from build123d import *

# Parameters (mm, degrees)
SKETCH1_R             = 5.715
BOSS_EXTRUDE1_DEPTH   = 76.2
SKETCH4_R             = 5.715
SKETCH4_R_2           = 5.207
BOSS_EXTRUDE2_DEPTH   = 3.81
F_6_32_TAPPED_HOLE1_D = 2.7051


with BuildPart() as part:
    # Sketch1 → Boss-Extrude1 (new body)
    with BuildSketch(Plane(origin=(0, 0, 0), x_dir=(1, 0, 0), z_dir=(0, 1, 0))):
        with BuildLine():
            Line((0, 8.255), (-10.795, 8.255))
            Line((-10.795, 8.255), (-10.795, -8.255))
            Line((-10.795, -8.255), (0, -8.255))
            ThreePointArc((0, -8.255), (8.255, 0), (0, 8.255))
        make_face()
        with Locations(Location((0, 0, 0), (0, 0, 90))):
            Circle(SKETCH1_R, mode=Mode.SUBTRACT)
    extrude(amount=BOSS_EXTRUDE1_DEPTH)

    # Sketch4 → Boss-Extrude2 (add)
    with BuildSketch(Plane.XZ):
        with Locations(Location((0, 0, 0), (0, 0, 270))):
            Circle(SKETCH4_R)
        with Locations(Location((0, 0, 0), (0, 0, 270))):
            Circle(SKETCH4_R_2, mode=Mode.SUBTRACT)
    extrude(amount=-BOSS_EXTRUDE2_DEPTH)

    # #6-32 Tapped Hole1 (through all)
    with Locations(Plane.ZY.offset(10.795)):
        with Locations((0, 69.85)):
            Hole(F_6_32_TAPPED_HOLE1_D / 2)


solid = part.part
The model under review builds one solid part; all positions refer to its coordinate system, in mm. A direction names the side the tool comes from. Give positions to 0.01 mm unless a question says otherwise; leave off trailing zeros. Order: outer loops, then holes, each group sorted by start corner. A loop starts at its lowest first (then second) coordinate and runs counter-clockwise, first axis right, second up. Notation, with made-up numbers: M -25.5,72.25 L 21.5,72.25 A12 cw 21.5,78.25 Z; hole C 3.5,4.25 d3. An arc over 180 degrees is marked long. Answer in a Markdown table with one row per item. Add a question column.
1. Add section B-B on y = 12. State the section outline as (x, z) points (3 decimals), plus the area to 3 significant figures.
2. Add section C-C on x = -1.25. State the section outline as (y, z) points (3 decimals), plus the area to 3 significant figures.
3. To check wall thickness, follow line 1 along X through (y, z) = (58.5, 0) (3 decimals); line 2 along Y through (x, z) = (-7, 0); line 3 along X through (y, z) = (1.3, 0) (3 decimals). State the ranges of each line that lie inside material, in increasing order.
4. Mouldability with a two-part tool opening along Z and no side actions: class faces 1 (the cylindrical face through (-5.666, 39.498, 0.744)), 2 (the flat face through (-5, 38, -8.255)), 3 (the flat face through (-5.4, 0, 0.1)) as released by +Z, released by -Z, zero draft, split by the parting line, or undercut.
5. Machinability: for faces 4 (the flat face through (-6, 76.2, -2)), 5 (the flat face through (-5, 3.81, -2)), which of the approach directions +Z, -Z, +X, -X, +Y, -Y give a long, thin tool a straight path to every point of the face, cutting with its end or side? Answer none if there is none.
6. Add section A-A on z = 0. State the section outline as (x, y) points (3 decimals).
7. Add section D-D on y = 69.85. State the section outline as (x, z) points (3 decimals).
8. For pin 1 Ø4 at (y, z) = (56.5, -4) entering from +X; pin 2 Ø6 at (x, z) = (0, 0) entering from -Y, all flat-tipped, find the tip position at first contact; note any pin that passes through.
The answers:
| question | item | result |
|---|---|---|
| 1 | outline | M -10.795,-8.255 L 0,-8.255 A8.255 ccw 0,8.255 L -10.795,8.255 Z; hole C 0,0 d11.43 |
| 1 | area | 183 mm2 |
| 2 | outline | M 0,-8.255 L 76.2,-8.255 L 76.2,-5.577 L 3.81,-5.577 L 3.81,-5.055 L 0,-5.055 Z; M 0,5.055 L 3.81,5.055 L 3.81,5.577 L 76.2,5.577 L 76.2,8.255 L 0,8.255 Z |
| 2 | area | 412 mm2 |
| 3 | line 1 | -10.795 to -5.715, 5.715 to 8.255 |
| 3 | line 2 | 0 to 68.5, 71.2 to 76.2 |
| 3 | line 3 | -10.795 to -5.207, 5.207 to 8.255 |
| 4 | face 1 | undercut |
| 4 | face 2 | released by -Z |
| 4 | face 3 | zero draft |
| 5 | face 4 | +Z, -Z, +X, -X, +Y |
| 5 | face 5 | +Y |
| 6 | outline | M -10.795,0 L -5.207,0 L -5.207,3.81 L -5.715,3.81 L -5.715,68.497 L -10.795,68.497 Z; M -10.795,71.203 L -5.715,71.203 L -5.715,76.2 L -10.795,76.2 Z; M 5.207,0 L 8.255,0 L 8.255,68.497 L 5.715,68.497 L 5.715,3.81 L 5.207,3.81 Z; M 5.715,71.203 L 8.255,71.203 L 8.255,76.2 L 5.715,76.2 Z |
| 7 | outline | M -10.795,-8.255 L 0,-8.255 A8.255 ccw 8.143,-1.353 L 5.553,-1.353 A5.715 cw -5.553,-1.353 L -10.795,-1.353 Z; M -10.795,1.353 L -5.553,1.353 A5.715 cw 5.553,1.353 L 8.143,1.353 A8.255 ccw 0,8.255 L -10.795,8.255 Z |
| 8 | pin 1 | x = 8.01 |
| 8 | pin 2 | through |
